The model under review builds one solid part; all positions refer to its coordinate system, in mm. Face numbers are marked on the shaded views. A direction names the side the tool comes from. Round coordinates to 2 decimals unless told otherwise and drop trailing zeros. Write each loop counter-clockwise with the first axis right and the second up, starting at its lowest first coordinate (ties: lowest second). Pieces come first, ordered by that corner, then holes. Notation, with made-up numbers: (-34, 16.5) - (20, 16.5) arc R19 cw to (20, 24.5) - close; hole circle Ø7 at (47.5, 20.5). An arc over 180 degrees is marked (long way). Write each question's results on one line, items separated by ' | '.
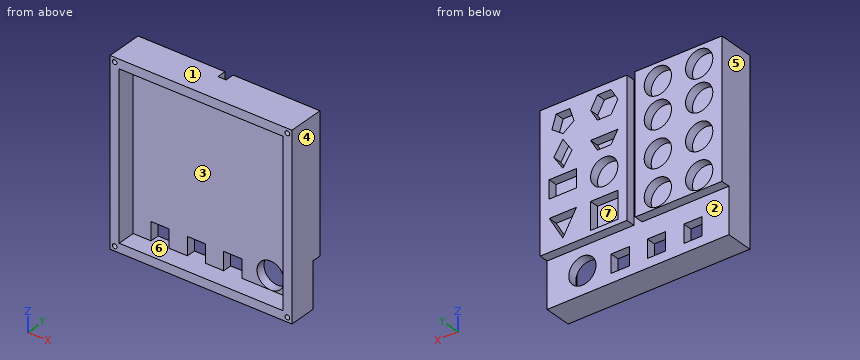
```python
from build123d import *

# Parameters (mm, degrees)
CROQUIS1_W              = 200
CROQUIS1_H              = 200
SALIENTE_EXTRUIR1_DEPTH = 10
CROQUIS2_W              = 95.5
CROQUIS2_H              = 150
SALIENTE_EXTRUIR2_DEPTH = 10
CROQUIS3_R              = 15
CROQUIS3_W              = 20
CROQUIS3_H              = 20
CORTAR_EXTRUIR1_DEPTH   = 284.019433962
CROQUIS4_W              = 200
CROQUIS4_H              = 200
CROQUIS4_W_2            = 180
CROQUIS4_H_2            = 180
SALIENTE_EXTRUIR3_DEPTH = 20
CROQUIS6_R              = 2.5
CORTAR_EXTRUIR2_DEPTH   = 15
CROQUIS7_R              = 15
CORTAR_EXTRUIR3_DEPTH   = 10
CROQUIS8_R              = 15
CROQUIS8_W              = 30
CROQUIS8_H              = 30
CROQUIS8_H_2            = 20
CORTAR_EXTRUIR4_DEPTH   = 10


with BuildPart() as part:
    # Croquis1 → Saliente-Extruir1 (new body)
    with BuildSketch(Plane(origin=(0, 0, 0), x_dir=(1, 0, 0), z_dir=(0, 1, 0))):
        with Locations((-100, 100)):
            Rectangle(CROQUIS1_W, CROQUIS1_H)
    extrude(amount=SALIENTE_EXTRUIR1_DEPTH)

    # Croquis2 → Saliente-Extruir2 (add)
    with BuildSketch(Plane(origin=(0, 10, 0), x_dir=(1, 0, 0), z_dir=(0, 1, 0))):
        with Locations((-47.75, 75)):
            Rectangle(CROQUIS2_W, CROQUIS2_H)
        with Locations((-152.25, 75)):
            Rectangle(CROQUIS2_W, CROQUIS2_H)
    extrude(amount=SALIENTE_EXTRUIR2_DEPTH)

    # Croquis3 → Cortar-Extruir1 (cut, through all)
    with BuildSketch(Plane(origin=(0, 10, 0), x_dir=(1, 0, 0), z_dir=(0, 1, 0))):
        with Locations(Location((-38.780765976, 175, 0), (0, 0, 270))):
            Circle(CROQUIS3_R)
        with Locations((-160.375957062, 180)):
            Rectangle(CROQUIS3_W, CROQUIS3_H)
        with Locations((-120.375957062, 180)):
            Rectangle(CROQUIS3_W, CROQUIS3_H)
        with Locations((-80.375957062, 180)):
            Rectangle(CROQUIS3_W, CROQUIS3_H)
    extrude(amount=-CORTAR_EXTRUIR1_DEPTH, mode=Mode.SUBTRACT)

    # Croquis4 → Saliente-Extruir3 (add)
    with BuildSketch(Plane(origin=(0, 0, 0), x_dir=(-1, 0, 0), z_dir=(0, -1, 0))):
        with Locations((100, 100)):
            Rectangle(CROQUIS4_W, CROQUIS4_H)
        with Locations((100, 100)):
            Rectangle(CROQUIS4_W_2, CROQUIS4_H_2, mode=Mode.SUBTRACT)
    extrude(amount=SALIENTE_EXTRUIR3_DEPTH)

    # Croquis6 → Cortar-Extruir2 (cut)
    with BuildSketch(Plane(origin=(0, -20, 0), x_dir=(-1, 0, 0), z_dir=(0, -1, 0))):
        with Locations(Location((195, 5, 0), (0, 0, 90))):
            Circle(CROQUIS6_R)
        with Locations(Location((5, 5, 0), (0, 0, 90))):
            Circle(CROQUIS6_R)
        with Locations(Location((5, 195, 0), (0, 0, 90))):
            Circle(CROQUIS6_R)
        with Locations(Location((195, 195, 0), (0, 0, 90))):
            Circle(CROQUIS6_R)
    extrude(amount=-CORTAR_EXTRUIR2_DEPTH, mode=Mode.SUBTRACT)

    # Croquis7 → Cortar-Extruir3 (cut)
    with BuildSketch(Plane(origin=(0, 20, 0), x_dir=(1, 0, 0), z_dir=(0, 1, 0))):
        with Locations(Location((-175, 134, 0), (0, 0, 270))):
            Circle(CROQUIS7_R)
        with Locations(Location((-129.5, 134, 0), (0, 0, 270))):
            Circle(CROQUIS7_R)
        with Locations(Location((-175, 94, 0), (0, 0, 270))):
            Circle(CROQUIS7_R)
        with Locations(Location((-129.5, 94, 0), (0, 0, 270))):
            Circle(CROQUIS7_R)
        with Locations(Location((-175, 54, 0), (0, 0, 270))):
            Circle(CROQUIS7_R)
        with Locations(Location((-129.5, 54, 0), (0, 0, 270))):
            Circle(CROQUIS7_R)
        with Locations(Location((-175, 19, 0), (0, 0, 270))):
            Circle(CROQUIS7_R)
        with Locations(Location((-129.5, 19, 0), (0, 0, 270))):
            Circle(CROQUIS7_R)
    extrude(amount=-CORTAR_EXTRUIR3_DEPTH, mode=Mode.SUBTRACT)

    # Croquis8 → Cortar-Extruir4 (cut)
    with BuildSketch(Plane(origin=(0, 20, 0), x_dir=(1, 0, 0), z_dir=(0, 1, 0))):
        with Locations(Location((-70.5, 90, 0), (0, 0, 270))):
            Circle(CROQUIS8_R)
        with Locations((-70.5, 130)):
            Rectangle(CROQUIS8_W, CROQUIS8_H)
        Polygon((-40, 115), (-10, 115), (-25, 140.980762114), align=None)
        Polygon((-85.5, 52.009587992), (-55.5, 52.009587992), (-63.049173048, 65.016851393), (-78.04913439, 64.982796557), align=None)
        with Locations((-25, 85)):
            Rectangle(CROQUIS8_W, CROQUIS8_H_2)
        Polygon((-25, 68.896042606), (-35, 53.896042606), (-25, 38.905718571), (-15, 53.896042606), align=None)
        Polygon((-55.5, 21.068183762), (-63, 34.058564819), (-78, 34.058564819), (-85.5, 21.068183762), (-78, 8.077802706), (-63, 8.077802706), align=None)
        Polygon((-25.135254916, 33.338916583), (-37.270509831, 24.522137799), (-32.635254916, 10.256290054), (-17.635254916, 10.256290054), (-13, 24.522137799), align=None)
    extrude(amount=-CORTAR_EXTRUIR4_DEPTH, mode=Mode.SUBTRACT)


solid = part.part
```
Q1. Tool access review of the marked faces 5, 6 and 7: name each direction out of +Z, -Z, +X, -X, +Y, -Y from which nothing blocks a thin tool from reaching the whole face with its end or side.
Evaluation:
face 5: +Z, -Z, -X, +Y, -Y | face 6: -Y | face 7: +Y
Q2. We need section A-A (x = -156.5). State the section outline as (y, z) points.
Evaluation:
outline: (-20, -200) - (10, -200) - (10, -190) - (-20, -190) - close; (-20, -10) - (0, -10) - (0, -170) - (10, -170) - (10, -150) - (20, -150) - (20, 0) - (-20, 0) - close
Q3. We need section C-C (z = -175). State the section outline as (x, y) points.
Evaluation:
outline: (-200, -20) - (-190, -20) - (-190, 0) - (-170.38, 0) - (-170.38, 10) - (-200, 10) - close; (-150.38, 0) - (-130.38, 0) - (-130.38, 10) - (-150.38, 10) - close; (-110.38, 0) - (-90.38, 0) - (-90.38, 10) - (-110.38, 10) - close; (-70.38, 0) - (-53.78, 0) - (-53.78, 10) - (-70.38, 10) - close; (-23.78, 0) - (-10, 0) - (-10, -20) - (0, -20) - (0, 10) - (-23.78, 10) - close
Q4. For probe 1 along X at (y, z) = (-12.75, -195); probe 2 along Z at (x, y) = (-129, 15), list the stretches that pass through material, from the lowest coordinate up.
Evaluation:
probe 1: x = -200 to -197.5, -192.5 to -7.5, -2.5 to 0 | probe 2: z = -150 to -148.99, -119.01 to -108.99, -79.01 to -68.99, -39.01 to -33.99, -4.01 to 0
Q5. We need section B-B (y = -15.5). State the section outline as (x, z) points, plus the area to 3 significant figures.
Evaluation:
outline: (-200, -200) - (0, -200) - (0, 0) - (-200, 0) - close; hole circle Ø5 at (-195, -195); hole circle Ø5 at (-195, -5); hole (-190, -190) - (-10, -190) - (-10, -10) - (-190, -10) - close; hole circle Ø5 at (-5, -195); hole circle Ø5 at (-5, -5) | area: 7,520 mm^2
Q6. The part is to be moulded in two halves that separate along X. For the marked faces 1, 2, 3 and 4, say which applies: released by +X, released by -X, zero draft, split by the parting line, or undercut.
Evaluation:
face 1: zero draft | face 2: undercut | face 3: undercut | face 4: released by +X
Q7. Insertion check: P1, Ø8, axis at x = -95.5, z = -144, coming from the -Y side; P2, Ø5, axis at x = -26, y = 15, coming from the -Z side; P3, Ø2.5, axis at x = -5, z = -5, coming from the -Y side. Each pin has a flat end and moves straight along its axis. Give the tip position at first contact, or say it passes through.
Evaluation:
P1: stops at y = 0 | P2: stops at z = -150 | P3: stops at y = -5
Q8. We need section D-D (x = -107.5). State the section outline as (y, z) points.
Evaluation:
outline: (-20, -200) - (10, -200) - (10, -150) - (20, -150) - (20, 0) - (-20, 0) - (-20, -10) - (0, -10) - (0, -190) - (-20, -190) - close
